from build123d import *

# Parameters (mm, degrees)
F0_R     = 10
F0_W     = 32
F0_H     = 1.5
F1_DEPTH = 23
F2_R     = 2.5
F3_DEPTH = 2
F4_R     = 2
F5_DEPTH = 10
F6_W     = 12
F6_H     = 12
F7_DEPTH = 2


with BuildPart() as f1:
    # F0 (on Front) → F1 (new body)
    with BuildSketch(Plane.XZ):
        with Locations((0, 12)):
            Circle(F0_R)
        with Locations((0, 0.75)):
            Rectangle(F0_W, F0_H)
    extrude(amount=F1_DEPTH)

    # F2 (on face) → F3 (join)
    with BuildSketch(Plane.XZ.offset(23)):
        with Locations((0, 12)):
            Circle(F2_R)
    extrude(amount=F3_DEPTH)

    # F4 (on face) → F5 (join)
    with BuildSketch(Plane.XZ.offset(25)):
        with Locations((0, 12)):
            Circle(F4_R)
    extrude(amount=F5_DEPTH)

    # F6 (on face) → F7 (join)
    with BuildSketch(Plane(origin=(0, 0, 0), x_dir=(-1, 0, 0), z_dir=(0, 1, 0))):
        with BuildLine():
            ThreePointArc((6, 12), (0, 18), (-6, 12))
            Line((-6, 12), (6, 12))
        make_face()
        with Locations((0, 6)):
            Rectangle(F6_W, F6_H)
    extrude(amount=F7_DEPTH)


solid = f1.part
Check sheet for the modelled part. Datum: model origin and axes. Units: mm. A direction names the side the tool comes from. Round coordinates to 2 decimals unless told otherwise and drop trailing zeros. Order: outer loops, then holes, each group sorted by start corner. A loop starts at its lowest first (then second) coordinate and runs counter-clockwise, first axis right, second up.
(1) Scan lines: probe 1 along Z at (x, y) = (0, -5); probe 2 along Y at (x, z) = (7.5, 11.75); probe 3 along Z at (x, y) = (-3.5, -9). Record each from-to range of solid material in increasing order.
(2) Cross-section at B-B, the plane x = 0. Enter the section's corners in (y, z), and give its area (4 significant figures).
(3) Cross-section at C-C, the plane z = 16.5. Enter the section's corners in (x, y).
(4) Go/stop test with flat-tipped pins: P1, Ø4, axis at y = -17.5, z = 6, coming from the -X side; P2, Ø2, axis at y = 1, z = 3.5, coming from the -X side; P3, Ø12, axis at x = -5, y = -20.5, coming from the -Z side; P4, Ø8, axis at x = -10, y = -20, coming from the +Z side. Record where each tip stops, or that it passes through.
(5) Access from +Z, -Z, +X, -X, +Y, -Y to the whole of each face (thin tool, end or side, straight path). Record for faces 1 (the flat face through (0, -11, 1.5)), 2 (the cylindrical face through (-2.17, -11.34, 2.24)), 3 (the flat face through (11, 0, 1)), 4 (the flat face through (0, 0, 19)), 5 (the flat face through (-11, 0, 1)).
(6) Cross-section at A-A, the plane y = -10.5. Enter the section's corners in (x, z), and give its area (3 significant figures).
(7) Cross-section at D-D, the plane z = 3. Enter the section's corners in (x, y), and give its area (3 significant figures).
Check sheet entries:
1. probe 1: z = 0 to 1.5, 2 to 22
1. probe 2: y = -23 to 0
1. probe 3: z = 0 to 1.5, 2.63 to 21.37
2. outline: (-35, 10) - (-25, 10) - (-25, 9.5) - (-23, 9.5) - (-23, 2) - (0, 2) - (0, 1.5) - (-23, 1.5) - (-23, 0) - (2, 0) - (2, 18) - (0, 18) - (0, 22) - (-23, 22) - (-23, 14.5) - (-25, 14.5) - (-25, 14) - (-35, 14) - close
2. area: 580.5 mm2
3. outline: (-8.93, -23) - (8.93, -23) - (8.93, 0) - (3.97, 0) - (3.97, 2) - (-3.97, 2) - (-3.97, 0) - (-8.93, 0) - close
4. P1: stops at x = -9.17
4. P2: stops at x = -6
4. P3: stops at z = 0
4. P4: stops at z = 20
5. face 1: +X, -X, -Y
5. face 2: -Y
5. face 3: +Z, -Z, +X, +Y
5. face 4: +Z, +Y
5. face 5: +Z, -Z, -X, +Y
6. outline: (-16, 0) - (16, 0) - (16, 1.5) - (-16, 1.5) - close; circle Ø20 at (0, 12)
6. area: 362 mm2
7. outline: (-6, 0) - (-4.36, 0) - (-4.36, -23) - (4.36, -23) - (4.36, 0) - (6, 0) - (6, 2) - (-6, 2) - close
7. area: 225 mm2
